```python
from build123d import *

# Parameters (mm, degrees)
F0_W     = 305
F0_H     = 210
F0_W_2   = 261
F0_H_2   = 166
F1_DEPTH = 3
F2_R     = 1
F3_R     = 1
F4_R     = 2.5
F5_DEPTH = 3


with BuildPart() as f1:
    # F0 (on Front) → F1 (new body)
    with BuildSketch(Plane.XZ):
        Rectangle(F0_W, F0_H)
        Rectangle(F0_W_2, F0_H_2, mode=Mode.SUBTRACT)
    extrude(amount=F1_DEPTH)

    # F2
    f2_edges = [f1.edges().sort_by_distance(p)[0] for p in [
        (-152.5, -1.5, 105),
        (-152.5, -1.5, -105),
        (152.5, -1.5, -105),
        (152.5, -1.5, 105),
    ]]
    fillet(f2_edges, radius=F2_R)

    # F3
    f3_edges = [f1.edges().sort_by_distance(p)[0] for p in [
        (0, -3, -105),
        (0, 0, -105),
    ]]
    fillet(f3_edges, radius=F3_R)

    # F4 (on face) → F5 (cut, through all)
    with BuildSketch(Plane.XZ.offset(3)):
        with Locations((-147.5, 100)):
            Circle(F4_R)
        with Locations((147.5, 100)):
            Circle(F4_R)
        with Locations((147.5, -100)):
            Circle(F4_R)
        with Locations((-147.5, -100)):
            Circle(F4_R)
    extrude(amount=-F5_DEPTH, mode=Mode.SUBTRACT)


solid = f1.part
```
The model under review builds one solid part; all positions refer to its coordinate system, in mm. Coordinates: 2 decimals unless noted, no trailing zeros. Order: outer loops, then holes, each group sorted by start corner. A loop starts at its lowest first (then second) coordinate and runs counter-clockwise, first axis right, second up. Notation, with made-up numbers: (83, 25.25) -> (117, 25.25) arc R29 ccw to (117, 54.25) -> close; hole circle Ø5 at (-29, -12.75). An arc over 180 degrees is marked (long way). Answer in a Markdown table with one row per item. Add a question column.
Item 1: Clearance check with a flat-ended pin moving along its axis: pin 1 (6.5 mm diameter, centred on x = -147.5, z = 100, fed in from +Y). State where the tip first meets the part, or that it passes through.
Item 2: We need section B-B on z = 25. Write out the cut boundary in (x, y), plus the area to 3 significant figures.
Item 3: To check wall thickness, follow probe 1 along Z at (x, y) = (-147.5, -1.85); probe 2 along X at (y, z) = (-1.2, -45); probe 3 along Z at (x, y) = (147.5, -2.4). State the ranges of each line that lie inside material, in increasing order.
Item 4: We need section A-A on x = -113.5. Write out the cut boundary in (y, z), plus the area to 3 significant figures.
Final values:
| question | item | result |
|---|---|---|
| 1 | pin 1 | stops at y = 0 |
| 2 | outline | (-152.5, -2) arc R1 ccw to (-151.5, -3) -> (-130.5, -3) -> (-130.5, 0) -> (-151.5, 0) arc R1 ccw to (-152.5, -1) -> close; (130.5, -3) -> (151.5, -3) arc R1 ccw to (152.5, -2) -> (152.5, -1) arc R1 ccw to (151.5, 0) -> (130.5, 0) -> close |
| 2 | area | 131 mm2 |
| 3 | probe 1 | z = -105 to -102.5, -97.5 to 97.5, 102.5 to 105 |
| 3 | probe 2 | x = -152.5 to -130.5, 130.5 to 152.5 |
| 3 | probe 3 | z = -104.92 to -102.5, -97.5 to 97.5, 102.5 to 104.92 |
| 4 | outline | (-3, -104) arc R1 ccw to (-2, -105) -> (-1, -105) arc R1 ccw to (0, -104) -> (0, -83) -> (-3, -83) -> close; (-3, 83) -> (0, 83) -> (0, 104) arc R1 ccw to (-1, 105) -> (-2, 105) arc R1 ccw to (-3, 104) -> close |
| 4 | area | 131 mm2 |
